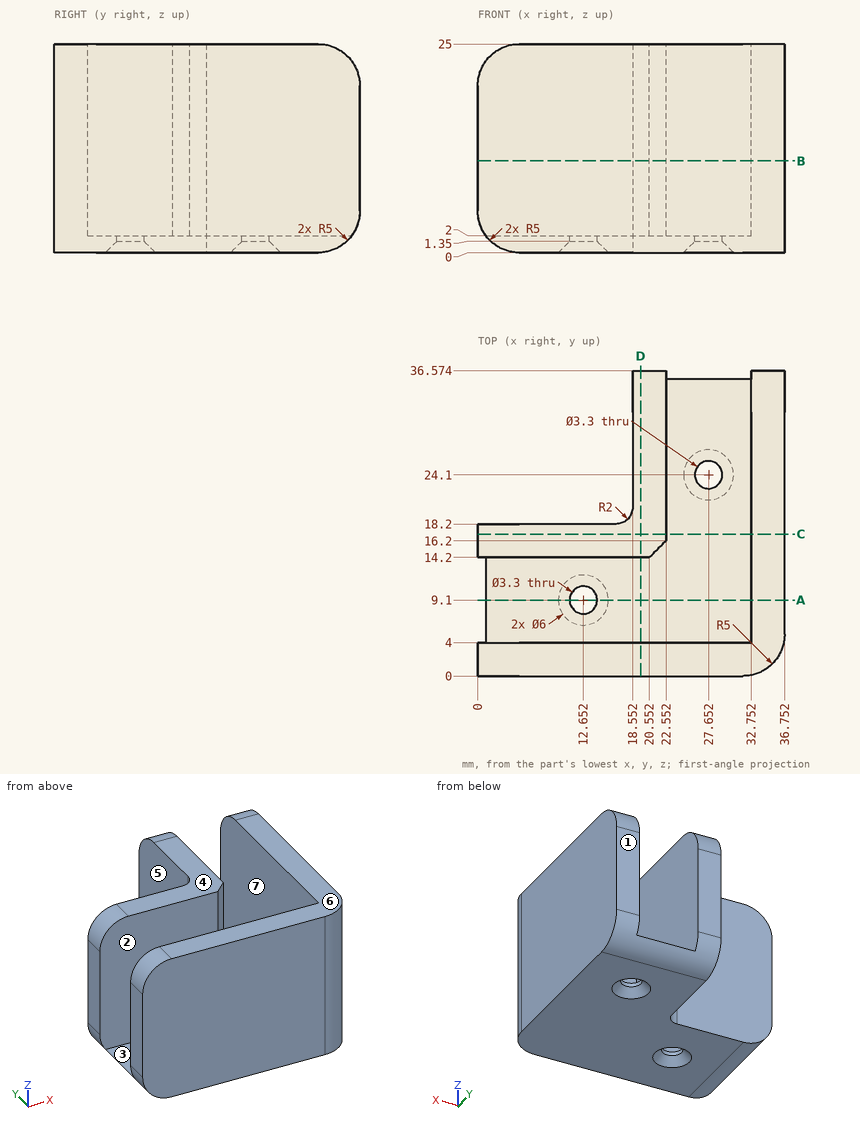
Here's the drawing with two shaded views (mm, measured from the low corner). I have some questions. A direction names the side the tool comes from. Coordinates: 2 decimals unless noted, no trailing zeros. Write each loop counter-clockwise with the first axis right and the second up, starting at its lowest first coordinate (ties: lowest second). Pieces come first, ordered by that corner, then holes. Notation, with made-up numbers: (39.25, 25) -> (92.25, 25) arc R33 cw to (92.25, 54) -> close; hole circle Ø2 at (62, 44.25). An arc over 180 degrees is marked (long way). Write item = value, one per line. Start each with the question number.
(1) We'd pull the mould along Y, two halves only. Please class the marked faces 1, 2, 3 and 4: released by +Y, released by -Y, zero draft, split by the parting line, or undercut.
(2) Which directions (+Z, -Z, +X, -X, +Y, -Y) give clear straight access to the entire face, cutting with the end or side of a thin tool? Please do the marked faces 5, 6 and 7.
(3) I want a section at D-D (x = 19.5). Please give me the cut outline in (y, z).
(4) I want a section at B-B (z = 11). Please give me the cut outline in (x, y).
(5) I want a section at C-C (y = 17). Please give me the cut outline in (x, z).
(6) Will these pins go through, and if not, where does the flat tip stop? pin 1 (8.5 mm diameter, centred on x = 8.5, z = 18, fed in from +Y); pin 2 (1.5 mm diameter, centred on y = 11, z = 5, fed in from -X); pin 3 (12 mm diameter, centred on y = 24.5, z = 9.5, fed in from -X) (1 decimal).
(7) I want a section at A-A (y = 9.1). Please give me the cut outline in (x, z), plus the area to 3 significant figures.
(8) I need wall thicknesses on line 1 (Y direction, x = 8, z = 21.5); line 2 (X direction, y = 30, z = 10.75); line 3 (X direction, y = 24.1, z = 1.6). Which ranges of each line are inside material? Lowest first, please. Write a range as [from, to].
Result set:
q1.face_1 = released by +Y
q1.face_2 = undercut
q1.face_3 = undercut
q1.face_4 = zero draft
q2.face_5 = +Z, -Z, -X, +Y
q2.face_6 = +Z, +X, -X, +Y, -Y
q2.face_7 = +Z, +Y
q3.outline = (0, 0) -> (31.57, 0) arc R5 ccw to (36.57, 5) -> (36.57, 20) arc R5 ccw to (31.57, 25) -> (14.2, 25) -> (14.2, 2) -> (4, 2) -> (4, 25) -> (0, 25) -> close
q4.outline = (0, 0) -> (31.75, 0) arc R5 ccw to (36.75, 5) -> (36.75, 36.57) -> (32.75, 36.57) -> (32.75, 4) -> (0, 4) -> close; (0, 14.2) -> (20.55, 14.2) -> (22.55, 16.2) -> (22.55, 36.57) -> (18.55, 36.57) -> (18.55, 20.2) arc R2 cw to (16.55, 18.2) -> (0, 18.2) -> close
q5.outline = (0, 5) arc R5 ccw to (5, 0) -> (36.75, 0) -> (36.75, 25) -> (32.75, 25) -> (32.75, 2) -> (22.55, 2) -> (22.55, 25) -> (5, 25) arc R5 ccw to (0, 20) -> close
q6.pin_1 = 18.2
q6.pin_2 = 32.75
q6.pin_3 = 17.6
q7.outline = (1, 2) arc R5 ccw to (5, 0) -> (9.65, 0) -> (11, 1.35) -> (11, 2) -> close; (14.3, 1.35) -> (15.65, 0) -> (36.75, 0) -> (36.75, 25) -> (32.75, 25) -> (32.75, 2) -> (14.3, 2) -> close
q7.area = 153 mm2
q8.line_1 = [0, 4], [14.2, 18.2]
q8.line_2 = [18.55, 22.55], [32.75, 36.75]
q8.line_3 = [18.55, 26], [29.3, 36.75]
